Read the model definition and answer for the solid it produces. Units are mm, in the model's axes. A direction names the side the tool comes from. Round coordinates to 2 decimals unless told otherwise and drop trailing zeros. Loops run counter-clockwise (first coordinate to the right, second up) from the corner with the lowest first, then second, coordinate; pieces in that order, holes last. Notation, with made-up numbers: M 30,19 L 35,19 A18 cw 35,51 Z; hole C 46.5,5 d1. An arc over 180 degrees is marked long. Write each question's results on one line, items separated by ' | '.
from build123d import *

# Parameters (mm, degrees)
F0_R      = 1.5
F1_DEPTH  = 6.9
F2_W      = 28.2
F2_H      = 73
F2_W_2    = 25.2
F2_H_2    = 63
F3_DEPTH  = 7
F4_R      = 5.75
F5_DEPTH  = 12.2727451706
F6_SIZE   = 2
F7_R      = 1.5
F8_DEPTH  = 3
F9_DEPTH  = 7.001
F10_DEPTH = 1.5


with BuildPart() as f1:
    # F0 (on Front) → F1 (new body, symmetric)
    with BuildSketch(Plane.XZ):
        with BuildLine():
            Line((-7, 2.7587302293), (-7, 0))
            Line((-7, 0), (7, 0))
            Line((7, 0), (7, 2))
            Line((7, 2), (10.8, 2))
            ThreePointArc((10.8, 2), (13.6348625345, 5.9816080739), (8.9448506986, 7.3576303929))
            ThreePointArc((8.9448506986, 7.3576303929), (-1.7475715563, 4.6720624952), (-10.8766435302, 10.8526946234))
            ThreePointArc((-10.8766435302, 10.8526946234), (-16.0476108736, 10.7307091252), (-13.4262707241, 6.2717451706))
            Line((-13.4262707241, 6.2717451706), (-11.7411403572, 6.2717451706))
            ThreePointArc((-11.7411403572, 6.2717451706), (-9.5241596378, 4.3079544417), (-7, 2.7587302293))
        make_face()
        with Locations((10.8, 5)):
            Circle(F0_R, mode=Mode.SUBTRACT)
        with Locations((-13.4262707241, 9.2717451706)):
            Circle(F0_R, mode=Mode.SUBTRACT)
    extrude(amount=F1_DEPTH, both=True)

    # F2 (on Right) → F3 (join, symmetric)
    with BuildSketch(Plane.YZ):
        with Locations((0, -33.5)):
            Rectangle(F2_W, F2_H)
        with Locations((0, -31.5)):
            Rectangle(F2_W_2, F2_H_2, mode=Mode.SUBTRACT)
    extrude(amount=F3_DEPTH, both=True)

    # F4 (on face) → F5 (cut, through all)
    with BuildSketch(Plane(origin=(0, 0, 0), x_dir=(1, 0, 0), z_dir=(0, 0, -1))):
        Circle(F4_R)
    extrude(amount=-F5_DEPTH, mode=Mode.SUBTRACT)

    # F6
    f6_edges = [f1.edges().sort_by_distance(p)[0] for p in [
        (0, -14.1, -70),
        (-7, 0, -70),
        (0, 14.1, -70),
        (7, 0, -70),
    ]]
    chamfer(f6_edges, length=F6_SIZE)

    # F7 (on face) → F8 (cut)
    with BuildSketch(Plane.XY.offset(-63)):
        with BuildLine():
            ThreePointArc((0, -5), (3.5355339059, -3.5355339059), (5, 0))
            ThreePointArc((5, 0), (3.5355339059, 3.5355339059), (0, 5))
            ThreePointArc((0, 5), (-5, 0), (0, -5))
        make_face()
        Circle(F7_R, mode=Mode.SUBTRACT)
    extrude(amount=-F8_DEPTH, mode=Mode.SUBTRACT)

    # F9 (cut, through all): a face of the model
    f9_faces = [f1.faces().sort_by_distance(p)[0] for p in [
        (0, 0, -63),
    ]]
    extrude(f9_faces, amount=-F9_DEPTH, mode=Mode.SUBTRACT)

    # F7 (on face) → F10 (cut)
    with BuildSketch(Plane.XY.offset(-63)):
        with BuildLine():
            ThreePointArc((0, 5), (3.5355339059, 3.5355339059), (5, 0))
            ThreePointArc((5, 0), (3.5355339059, -3.5355339059), (0, -5))
            Line((0, -5), (7, -5))
            Line((7, -5), (7, 5))
            Line((7, 5), (0, 5))
        make_face()
    extrude(amount=-F10_DEPTH, mode=Mode.SUBTRACT)


solid = f1.part
Item 1: The part is cut by section C-C (x = 3). Determine the outline of the cut face in (y, z), plus the area to 3 significant figures.
Outcome:
outline: M -14.1,-68 L -12.1,-70 L 12.1,-70 L 14.1,-68 L 14.1,3 L 6.9,3 L 6.9,4.68 L 4.91,4.68 L 4.91,0 L 12.6,0 L 12.6,-63 L 5,-63 L 5,-64.5 L 4,-64.5 L 4,-66 L -4,-66 L -4,-64.5 L -5,-64.5 L -5,-63 L -12.6,-63 L -12.6,0 L -4.91,0 L -4.91,4.68 L -6.9,4.68 L -6.9,3 L -14.1,3 Z | area: 417 mm2
Item 2: Flat-ended cylindrical pins translate along their axes: pin 1 (11 mm diameter, centred on x = 1.5, y = -3.5, fed in from +Z); pin 2 (1 mm diameter, centred on x = 5.5, y = -1, fed in from +Z); pin 3 (2 mm diameter, centred on x = 2, y = -11, fed in from +Z). Find the tip coordinate at first contact, or state that the pin passes through.
Outcome:
pin 1: stops at z = 6.08 | pin 2: stops at z = 5.6 | pin 3: stops at z = 3
Item 3: The part is cut by section D-D (x = 8). Determine the outline of the cut face in (y, z), plus the area to 3 significant figures.
Outcome:
outline: M -6.9,2 L 6.9,2 L 6.9,6.68 L -6.9,6.68 Z | area: 64.6 mm2
Item 4: The mould has two halves that part along Z. Classify faces 1 (the face through (-13, 0, 6.272)), 2 (the face through (0, -6, 0)), 3 (the face through (-3, -6.9, 4)), 4 (the face through (12.186, 0.097, 4.425)): pulls with the +Z half, pulls with the -Z half, needs draft (parallel to the pull), parting line crosses it, or undercut.
Outcome:
face 1: pulls with the -Z half | face 2: undercut | face 3: needs draft | face 4: undercut
Item 5: The part is cut by section A-A (y = 9). Determine the outline of the cut face in (x, z).
Outcome:
outline: M -7,-68 L -5,-70 L 5,-70 L 7,-68 L 7,-63 L -7,-63 Z; M -7,0 L 7,0 L 7,3 L -7,3 Z
Item 6: The part is cut by section B-B (z = -12). Determine the outline of the cut face in (x, y), plus the area to 3 significant figures.
Outcome:
outline: M -7,-14.1 L 7,-14.1 L 7,-12.6 L -7,-12.6 Z; M -7,12.6 L 7,12.6 L 7,14.1 L -7,14.1 Z | area: 42.0 mm2
Item 7: Straight lines are drawn through the part: line 1 (Z direction, x = 4, y = -9.75); line 2 (Y direction, x = 3.5, z = -52); line 3 (Y direction, x = 0, z = -67.6). For each, find the intervals that lie inside material, in ascending order.
Outcome:
line 1: z = -70 to -63, 0 to 3 | line 2: y = -14.1 to -12.6, 12.6 to 14.1 | line 3: y = -14.1 to -1.5, 1.5 to 14.1
Item 8: For faces 5 (the face through (0, 12.6, -32)), 6 (the face through (3, -5, -64)), 7 (the face through (13.66, -0.1, 5.91)), 8 (the face through (0, 10, 3)), 9 (the face through (-0.1, -13.1, -69)), determine the directions among +Z, -Z, +X, -X, +Y, -Y from which every point of the face is accessible in a straight line to the end or side of a thin tool.
Outcome:
face 5: +X, -X | face 6: +X | face 7: +Y, -Y | face 8: +Z, +X, -X, +Y | face 9: -Z, +X, -X, -Y
